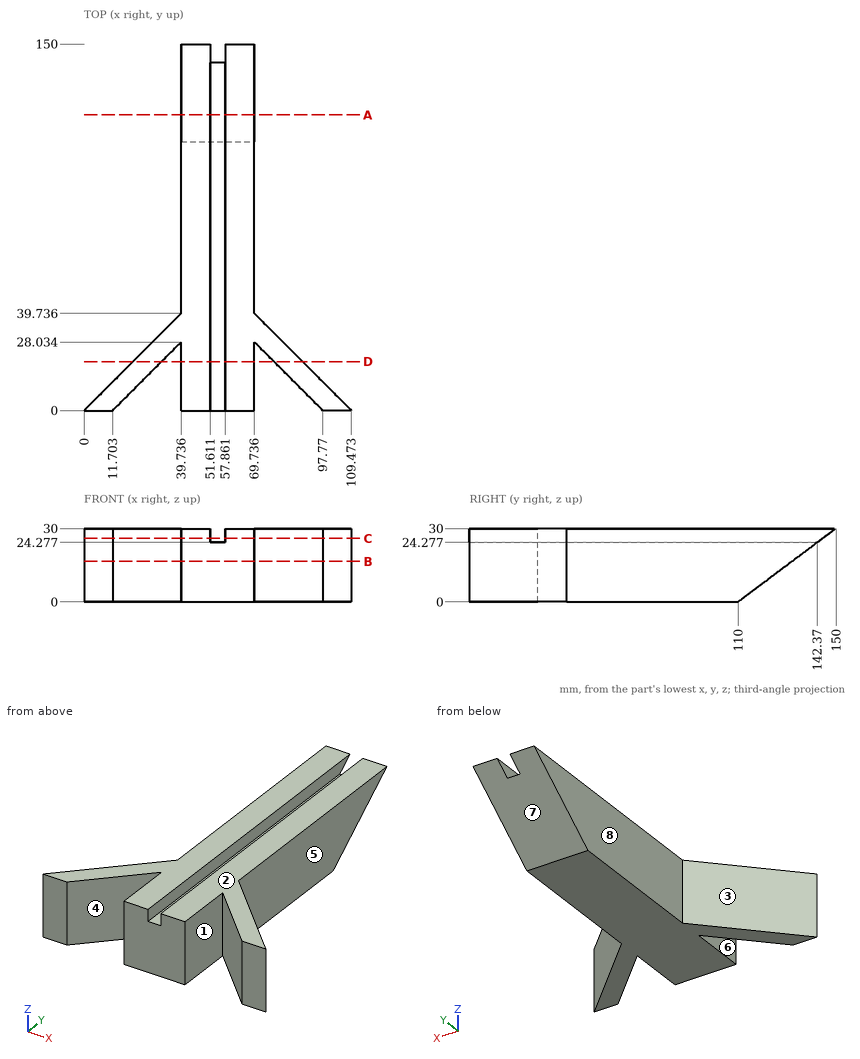
Verification items for this drawing (mm, ordinates from the low corner). A direction names the side the tool comes from. Coordinates: 2 decimals unless noted, no trailing zeros. Loops run counter-clockwise (first coordinate to the right, second up) from the corner with the lowest first, then second, coordinate; pieces in that order, holes last.
Item 1: Sectioned sample at A-A, the plane y = 121. Record the boundary of the cut face in (x, z), then the cut area to 3 significant figures.
Item 2: Sectioned sample at C-C, the plane z = 26. Record the boundary of the cut face in (x, y), then the cut area to 3 significant figures.
Item 3: Go/stop test with flat-tipped pins: pin 1 Ø6.5 at (y, z) = (53.5, 26.5) entering from -X; pin 2 Ø2 at (x, y) = (39.5, 119.5) entering from +Z; pin 3 Ø4 at (x, z) = (18, 7.5) entering from -Y; pin 4 Ø2 at (y, z) = (46.5, 14.5) entering from +X. Record where each tip stops, or that it passes through.
Item 4: Release check for a two-part mould opening along X. For the marked faces 1, 2, 3 and 4 record: released by +X, released by -X, zero draft, split by the parting line, or undercut.
Item 5: Access from +Z, -Z, +X, -X, +Y, -Y to the whole of each face (thin tool, end or side, straight path). Record for the marked faces 5, 6, 7 and 8.
Item 6: Thickness scan on line 1 (X direction, y = 26, z = 26.25) (1 decimal); line 2 (X direction, y = 41.5, z = 26); line 3 (X direction, y = 92, z = 16). Record the ranges inside material, lowest first.
Item 7: Sectioned sample at B-B, the plane z = 16.5. Record the boundary of the cut face in (x, y), then the cut area to 3 significant figures.
Item 8: Sectioned sample at D-D, the plane y = 20. Record the boundary of the cut face in (x, z), then the cut area to 3 significant figures.
Check result:
1. outline: (39.74, 8.25) - (69.74, 8.25) - (69.74, 30) - (57.86, 30) - (57.86, 24.28) - (51.61, 24.28) - (51.61, 30) - (39.74, 30) - close
1. area: 617 mm2
2. outline: (0, 0) - (11.7, 0) - (39.74, 28.03) - (39.74, 0) - (51.61, 0) - (51.61, 144.67) - (39.74, 144.67) - (39.74, 39.74) - close; (57.86, 0) - (69.74, 0) - (69.74, 28.03) - (97.77, 0) - (109.47, 0) - (69.74, 39.74) - (69.74, 144.67) - (57.86, 144.67) - close
2. area: 4,230 mm2
3. pin 1: stops at x = 39.74
3. pin 2: stops at z = 30
3. pin 3: stops at y = 4.3
3. pin 4: stops at x = 69.74
4. face 1: undercut
4. face 2: zero draft
4. face 3: released by -X
4. face 4: undercut
5. face 5: +Z, -Z, +X, +Y
5. face 6: +Z, -Z, -Y
5. face 7: -Z, +X, -X, +Y
5. face 8: +Z, -Z, -X, +Y
6. line 1: x = 26 to 37.7, 39.7 to 51.6, 57.9 to 69.7, 71.8 to 83.5
6. line 2: x = 39.74 to 51.61, 57.86 to 69.74
6. line 3: x = 39.74 to 69.74
7. outline: (0, 0) - (11.7, 0) - (39.74, 28.03) - (39.74, 0) - (69.74, 0) - (69.74, 28.03) - (97.77, 0) - (109.47, 0) - (69.74, 39.74) - (69.74, 132) - (39.74, 132) - (39.74, 39.74) - close
7. area: 4,750 mm2
8. outline: (20, 0) - (31.7, 0) - (31.7, 30) - (20, 30) - close; (39.74, 0) - (69.74, 0) - (69.74, 30) - (57.86, 30) - (57.86, 24.28) - (51.61, 24.28) - (51.61, 30) - (39.74, 30) - close; (77.77, 0) - (89.47, 0) - (89.47, 30) - (77.77, 30) - close
8. area: 1,570 mm2
